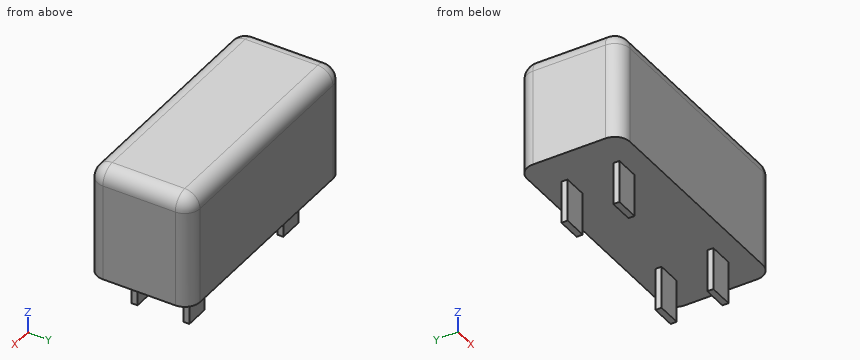
from build123d import *

# Parameters (mm, degrees)
SKETCH_W     = 16
SKETCH_H     = 6.75
PAD_DEPTH    = 7.37
SKETCH001_W  = 1.6
SKETCH001_H  = 0.4
PAD001_DEPTH = 2.8
FILLET_R     = 1


with BuildPart() as part:
    # Sketch → Pad (new body)
    with BuildSketch(Plane.XY):
        with Locations((8, 3.375)):
            Rectangle(SKETCH_W, SKETCH_H)
    extrude(amount=PAD_DEPTH)

    # Sketch001 → Pad001 (join)
    with BuildSketch(Plane.XY):
        with Locations((3.05, 5.075)):
            Rectangle(SKETCH001_W, SKETCH001_H)
        with Locations((12.95, 5.075)):
            Rectangle(SKETCH001_W, SKETCH001_H)
        with Locations((12.95, 1.675)):
            Rectangle(SKETCH001_W, SKETCH001_H)
        with Locations((3.05, 1.675)):
            Rectangle(SKETCH001_W, SKETCH001_H)
    extrude(amount=-PAD001_DEPTH)

    # Fillet
    fillet_edges = [part.edges().sort_by_distance(p)[0] for p in [
        (0, 0, 3.685),
        (8, 0, 7.37),
        (16, 3.375, 7.37),
        (8, 6.75, 7.37),
        (0, 3.375, 7.37),
        (16, 0, 3.685),
        (16, 6.75, 3.685),
        (0, 6.75, 3.685),
    ]]
    fillet(fillet_edges, radius=FILLET_R)


solid = part.part
Model file for the job. Use its own axes, mm. Give positions to 0.01 mm unless a question says otherwise; leave off trailing zeros. Order: outer loops, then holes, each group sorted by start corner. A loop starts at its lowest first (then second) coordinate and runs counter-clockwise, first axis right, second up. Notation, with made-up numbers: (44.25, 43.25) - (75.25, 43.25) arc R29 ccw to (75.25, 64.25) - close; hole circle Ø1 at (-3, 10.25). An arc over 180 degrees is marked (long way). One line per item, written item: value.
Item 1: Slice it at B-B (y = 4.5). List the corners of the cut face in (x, z), then the cut area to 3 significant figures.
Response values:
outline: (0, 0) - (16, 0) - (16, 6.37) arc R1 ccw to (15, 7.37) - (1, 7.37) arc R1 ccw to (0, 6.37) - close
area: 117 mm2
Item 2: Slice it at A-A (z = -2). List the corners of the cut face in (x, y) (3 decimals), then the cut area to 3 significant figures.
Response values:
outline: (2.25, 1.475) - (3.85, 1.475) - (3.85, 1.875) - (2.25, 1.875) - close; (2.25, 4.875) - (3.85, 4.875) - (3.85, 5.275) - (2.25, 5.275) - close; (12.15, 1.475) - (13.75, 1.475) - (13.75, 1.875) - (12.15, 1.875) - close; (12.15, 4.875) - (13.75, 4.875) - (13.75, 5.275) - (12.15, 5.275) - close
area: 2.56 mm2
Item 3: Slice it at C-C (x = 14.25). List the corners of the cut face in (y, z), then the cut area to 3 significant figures.
Response values:
outline: (0, 0) - (6.75, 0) - (6.75, 6.37) arc R1 ccw to (5.75, 7.37) - (1, 7.37) arc R1 ccw to (0, 6.37) - close
area: 49.3 mm2
Item 4: Slice it at D-D (z = 6.75). List the corners of the cut face in (x, y), then the cut area to 3 significant figures.
Response values:
outline: (0.08, 1) arc R0.92 ccw to (1, 0.08) - (15, 0.08) arc R0.92 ccw to (15.92, 1) - (15.92, 5.75) arc R0.92 ccw to (15, 6.67) - (1, 6.67) arc R0.92 ccw to (0.08, 5.75) - close
area: 104 mm2
Item 5: Pin check, flat tips, straight feed: pin 1 Ø1.8 at (x, z) = (3, -2) entering from +Y (3 decimals); pin 2 Ø1.8 at (x, z) = (3, -1) entering from -Y (3 decimals); pin 3 Ø2 at (x, y) = (2, 3) entering from -Z. Stop position of each tip, or through.
Response values:
pin 1: y = 5.275
pin 2: y = 1.475
pin 3: z = 0
Item 6: Wall check: line 1 (X direction, y = 1.75, z = -1.5); line 2 (Z direction, x = 9.5, y = 5.5); line 3 (Y direction, x = 12.75, z = -1) (3 decimals). Give the ranges that are in metal, low to high.
Response values:
line 1: 2.25 to 3.85, 12.15 to 13.75
line 2: 0 to 7.37
line 3: 1.475 to 1.875, 4.875 to 5.275
